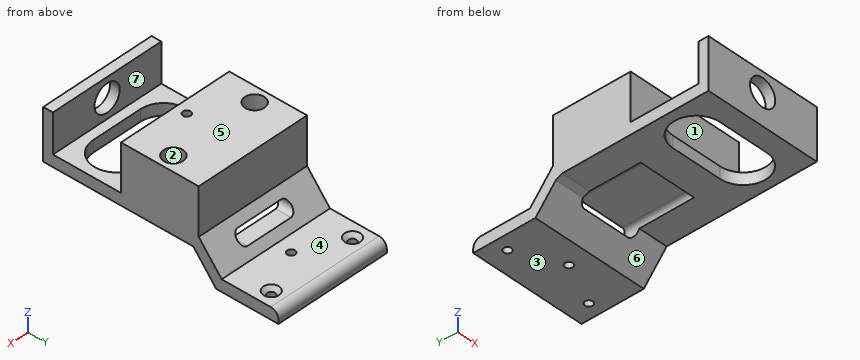
```python
from build123d import *

# Parameters (mm, degrees)
PAD005_DEPTH        = 15
SKETCH010_W         = 20
SKETCH010_H         = 30
SKETCH010_R         = 2.5
SKETCH010_R_2       = 1
PAD006_DEPTH        = 12
POCKET004_DEPTH     = 20
POCKET004_FACE013_W = 30
POCKET004_FACE013_H = 3
PAD010_DEPTH        = 20
SKETCH012_W         = 2.5
SKETCH012_H         = 30
PAD008_DEPTH        = 10
SKETCH013_R         = 3.5
POCKET005_DEPTH     = 5
POCKET006_DEPTH     = 5
SKETCH015_R         = 1
POCKET007_DEPTH     = 5
FILLET003_R         = 2
CHAMFER001_SIZE     = 1


with BuildPart() as part:
    # Sketch009 → Pad005 (new body, symmetric)
    with BuildSketch(Plane.YZ):
        Polygon((-53.6044145035, 7), (-59.4999553571, 14), (-79.4999553571, 14), (-79.4999553571, 11), (-60.8955408536, 11), (-55, 4), (-39, 4), (-39, 7), align=None)
    extrude(amount=PAD005_DEPTH, both=True)

    # Sketch010 (on Face5 of Pad005) → Pad006 (join)
    with BuildSketch(Plane(origin=(0, 0, 14), x_dir=(0, -1, 0), z_dir=(0, 0, 1))):
        with Locations((69.4999553571, 0)):
            Rectangle(SKETCH010_W, SKETCH010_H)
        with Locations((69.4999553571, 11.25)):
            Circle(SKETCH010_R, mode=Mode.SUBTRACT)
        with Locations((69.4999553571, -11.25)):
            Circle(SKETCH010_R, mode=Mode.SUBTRACT)
        with Locations((76.4999553571, 0)):
            Circle(SKETCH010_R_2, mode=Mode.SUBTRACT)
    extrude(amount=PAD006_DEPTH)

    # Sketch011 → Pocket004 (cut)
    with BuildSketch(Plane.XZ.offset(55)):
        with BuildLine():
            ThreePointArc((-6, 12), (-7.5, 10.5), (-6, 9))
            Line((-6, 9), (6, 9))
            ThreePointArc((6, 9), (7.5, 10.5), (6, 12))
            Line((6, 12), (-6, 12))
        make_face()
    extrude(amount=POCKET004_DEPTH, mode=Mode.SUBTRACT)

    # Pocket004 Face013 → Pad010 (add)
    with BuildSketch(Plane(origin=(0, -79.4999553571, 12.5), x_dir=(-1, 0, 0), z_dir=(0, -1, 0))):
        Rectangle(POCKET004_FACE013_W, POCKET004_FACE013_H)
    extrude(amount=PAD010_DEPTH)

    # Sketch012 (on Face22 of Pad010) → Pad008 (join)
    with BuildSketch(Plane(origin=(0, 0, 14), x_dir=(0, -1, 0), z_dir=(0, 0, 1))):
        with Locations((98.2499553571, 0)):
            Rectangle(SKETCH012_W, SKETCH012_H)
    extrude(amount=PAD008_DEPTH)

    # Sketch013 (on Face30 of Pad008) → Pocket005 (cut)
    with BuildSketch(Plane(origin=(0, -99.4999553571, 0), x_dir=(0, 0, -1), z_dir=(0, -1, 0))):
        with Locations((-19, 0)):
            Circle(SKETCH013_R)
    extrude(amount=-POCKET005_DEPTH, mode=Mode.SUBTRACT)

    # Sketch014 (on Face22 of Pocket005) → Pocket006 (cut)
    with BuildSketch(Plane(origin=(0, 0, 14), x_dir=(0, -1, 0), z_dir=(0, 0, 1))):
        with BuildLine():
            ThreePointArc((94.4999553571, 6.5), (88.4999553571, 12.5), (82.4999553571, 6.5))
            Line((82.4999553571, 6.5), (82.4999553571, -6.5))
            ThreePointArc((82.4999553571, -6.5), (88.4999553571, -12.5), (94.4999553571, -6.5))
            Line((94.4999553571, -6.5), (94.4999553571, 6.5))
        make_face()
    extrude(amount=-POCKET006_DEPTH, mode=Mode.SUBTRACT)

    # Sketch015 (on Face1 of Pocket006) → Pocket007 (cut)
    with BuildSketch(Plane.YX.offset(-4)):
        with Locations((-44.3333333333, 11.25)):
            Circle(SKETCH015_R)
        with Locations((-44.3333333333, -11.25)):
            Circle(SKETCH015_R)
        with Locations((-49.6666666667, 0)):
            Circle(SKETCH015_R)
    extrude(amount=-POCKET007_DEPTH, mode=Mode.SUBTRACT)

    # Fillet003
    fillet003_edges = [part.edges().sort_by_distance(p)[0] for p in [
        (0, -39, 7),
        (6, -66.407758, 12),
    ]]
    fillet(fillet003_edges, radius=FILLET003_R)

    # Chamfer001
    chamfer001_edges = [part.edges().sort_by_distance(p)[0] for p in [
        (-11.207107, -60.895541, 11),
        (-11.25, -45.333333, 7),
        (11.25, -45.333333, 7),
    ]]
    chamfer(chamfer001_edges, length=CHAMFER001_SIZE)


solid = part.part
```
Build history of the part. All positions in model axes, mm. Face numbers are marked on the shaded views. A direction names the side the tool comes from. Round coordinates to 2 decimals unless told otherwise and drop trailing zeros. Write each loop counter-clockwise with the first axis right and the second up, starting at its lowest first coordinate (ties: lowest second). Pieces come first, ordered by that corner, then holes.
1) Band-saw the part on C-C, the plane y = -65. List the corners of the cut face in (x, z), and give its area (3 significant figures).
2) 3-axis set-ups, long thin cutter, end or side, ignore diameter. For the marked faces 1, 2, 3 and 4: which of +Z, -Z, +X, -X, +Y, -Y reach the whole face in a straight line?
3) Drill centre lines: probe 1 along X at (y, z) = (-98.8, 19); probe 2 along Y at (x, z) = (13, 19.5); probe 3 along Y at (x, z) = (-3.5, 15.5). Where is each one in solid material? Low to high.
4) Band-saw the part on B-B, the plane x = 0. Give the number of separate pieces and of enclosed holes in the cut face, and give its area (3 significant figures).
5) Band-saw the part on D-D, the plane x = 11.25. List the corners of the cut face in (y, z).
6) Mould opens along Y. For the marked faces 5, 6 and 7 say: +Y half, -Y half, draft (parallel to the pull), parting line (faces both ways), or undercut.
7) Band-saw the part on A-A, the plane z = 19. List the corners of the cut face in (x, y), and give its area (3 significant figures).
8) Pin check, flat tips, straight feed: pin 1 (1.5 mm diameter, centred on y = -66, z = 9.5, fed in from +X); pin 2 (2 mm diameter, centred on x = -6, z = 20, fed in from +Y); pin 3 (0.9 mm diameter, centred on x = -3, z = 12, fed in from +Y); pin 4 (1.5 mm diameter, centred on x = 3.5, y = -45, fed in from +Z). Stop position of each tip, or through.
Ans:
1. outline: (-15, 11) - (-7.41, 11) arc R1.5 cw to (-6, 12) - (6, 12) arc R1.5 cw to (7.41, 11) - (15, 11) - (15, 26) - (-15, 26) - close
1. area: 436 mm2
2. face 1: +Z, +X, -X
2. face 2: +Z
2. face 3: -Z, +X, -X, +Y, -Y
2. face 4: +Z, +X, -X, +Y
3. probe 1: x = -15 to -3.5, 3.5 to 15
3. probe 2: y = -99.5 to -97, -79.5 to -71.29, -67.71 to -59.5
3. probe 3: y = -99.5 to -97, -79.5 to -59.5
4. separate pieces: 5
4. enclosed holes: 0
4. area: 346 mm2
5. outline: (-99.5, 11) - (-92.17, 11) - (-92.17, 14) - (-97, 14) - (-97, 24) - (-99.5, 24) - close; (-84.83, 11) - (-60.9, 11) - (-55, 4) - (-45.33, 4) - (-45.33, 6) - (-46.33, 7) - (-53.6, 7) - (-59.5, 14) - (-59.5, 26) - (-67, 26) - (-67, 14) - (-72, 14) - (-72, 26) - (-79.5, 26) - (-79.5, 14) - (-84.83, 14) - close; (-43.33, 4) - (-39, 4) - (-39, 5) arc R2 ccw to (-41, 7) - (-42.33, 7) - (-43.33, 6) - close
6. face 5: draft
6. face 6: -Y half
6. face 7: undercut
7. outline: (-15, -99.5) - (-3.5, -99.5) - (-3.5, -97) - (-15, -97) - close; (-15, -79.5) - (15, -79.5) - (15, -59.5) - (-15, -59.5) - close; (3.5, -99.5) - (15, -99.5) - (15, -97) - (3.5, -97) - close; hole circle Ø5 at (-11.25, -69.5); hole circle Ø2 at (0, -76.5); hole circle Ø5 at (11.25, -69.5)
7. area: 615 mm2
8. pin 1: passes through
8. pin 2: stops at y = -59.5
8. pin 3: stops at y = -57.82
8. pin 4: stops at z = 7
